Check sheet for the modelled part. Datum: model origin and axes. Units: mm. A direction names the side the tool comes from. Give positions to 0.01 mm unless a question says otherwise; leave off trailing zeros. Order: outer loops, then holes, each group sorted by start corner. A loop starts at its lowest first (then second) coordinate and runs counter-clockwise, first axis right, second up. Notation, with made-up numbers: M -34.5,87.25 L 8.5,87.25 A26 cw 8.5,109.25 Z; hole C 15.25,50 d7. An arc over 180 degrees is marked long. Return JSON: item names as keys, results as strings. Group by question number.
from build123d import *

# Parameters (mm, degrees)
BOSS_EXTRUDE2_DEPTH = 5.08
FILLET2_R           = 9.525
FILLET3_R           = 25.4


with BuildPart() as part:
    # Sketch5 → Boss-Extrude2 (new body)
    with BuildSketch(Plane(origin=(0, 0, -50.8), x_dir=(-1, 0, 0), z_dir=(0, 0, -1))):
        with BuildLine():
            Line((-52.084134713, -74.90469108), (-56.217901117, -96.079564574))
            ThreePointArc((-56.217901117, -96.079564574), (-56.227450796, -96.143111106), (-56.231425689, -96.207248133))
            Line((-56.231425689, -96.207248133), (-56.695270711, -121.603012501))
            Line((-56.695270711, -121.603012501), (-61.45697653, -121.516041559))
            Line((-61.45697653, -121.516041559), (-61.688899041, -134.213923743))
            Line((-61.688899041, -134.213923743), (-56.927193222, -134.300894684))
            Line((-56.927193222, -134.300894684), (-57.620624926, -172.266653317))
            Line((-57.620624926, -172.266653317), (-36.877249891, -96.432815008))
            Line((-36.877249891, -96.432815008), (19.109812826, -97.455399718))
            Line((19.109812826, -97.455399718), (37.101706355, -172.266653317))
            Line((37.101706355, -172.266653317), (37.763549432, -136.03038898))
            Line((37.763549432, -136.03038898), (42.525255251, -136.117359921))
            Line((42.525255251, -136.117359921), (42.757177762, -123.419477738))
            Line((42.757177762, -123.419477738), (37.995471943, -123.332506796))
            Line((37.995471943, -123.332506796), (38.459316965, -97.936742429))
            ThreePointArc((38.459316965, -97.936742429), (38.457686823, -97.872503028), (38.450464051, -97.808650153))
            Line((38.450464051, -97.808650153), (35.09270057, -76.496946406))
            Line((35.09270057, -76.496946406), (39.797167723, -75.755734526))
            Line((39.797167723, -75.755734526), (36.832320201, -56.937865912))
            Line((36.832320201, -56.937865912), (32.127853048, -57.679077792))
            Line((32.127853048, -57.679077792), (24.22159299, -7.498094822))
            ThreePointArc((24.22159299, -7.498094822), (23.977671585, -7.057207813), (23.507420242, -6.876258426))
            Line((23.507420242, -6.876258426), (11.818416858, -6.662762744))
            Line((11.818416858, -6.662762744), (11.905387799, -1.901056925))
            Line((11.905387799, -1.901056925), (-26.188258752, -1.205289392))
            Line((-26.188258752, -1.205289392), (-26.275229693, -5.966995211))
            Line((-26.275229693, -5.966995211), (-37.964233078, -5.753499529))
            ThreePointArc((-37.964233078, -5.753499529), (-38.44077853, -5.917155993), (-38.700637178, -6.348841631))
            Line((-38.700637178, -6.348841631), (-48.434089931, -56.20764123))
            Line((-48.434089931, -56.20764123), (-53.108352393, -55.295130035))
            Line((-53.108352393, -55.295130035), (-56.758397176, -73.992179884))
            Line((-56.758397176, -73.992179884), (-52.084134713, -74.90469108))
        make_face()
        Polygon((-31.935446416, -71.118839034), (-23.256774895, -26.66306829), (8.046213899, -27.234806762), (15.095699394, -71.977846959), align=None, mode=Mode.SUBTRACT)
    extrude(amount=BOSS_EXTRUDE2_DEPTH)

    # Fillet2
    fillet2_edges = [part.edges().sort_by_distance(p)[0] for p in [
        (31.935446416, -71.118839034, -53.34),
        (-15.095699394, -71.977846959, -53.34),
        (-8.046213899, -27.234806762, -53.34),
        (23.256774895, -26.66306829, -53.34),
    ]]
    fillet(fillet2_edges, radius=FILLET2_R)

    # Fillet3
    fillet3_edges = [part.edges().sort_by_distance(p)[0] for p in [
        (-19.109812826, -97.455399718, -53.34),
        (36.877249891, -96.432815008, -53.34),
    ]]
    fillet(fillet3_edges, radius=FILLET3_R)


solid = part.part
1) Release check for a two-part mould opening along X. For faces 1 (the face through (49.964, -144.275, -53.304)), 2 (the face through (10, -86, -50.8)), 3 (the face through (-38.335, -66.479, -53.304)) record: released by +X, released by -X, zero draft, split by the parting line, or undercut.
2) Sectioned sample at B-B on y = -52. Record the boundary of the cut face in (x, z), then the cut area to 3 significant figures.
3) Material ranges on line 1 along X through (y, z) = (-120.5, -53.05); line 2 along X through (y, z) = (-107.5, -51.95); line 3 along Y through (x, z) = (10, -51.9), recorded low to high.
4) Depth check by flat-ended pin: P1, Ø2, axis at x = 39.5, z = -52.5, coming from the -Y side; P2, Ø1, axis at x = -21.5, z = -55, coming from the +Y side. Enter the tip coordinate at first touch or a pass-through.
5) Sectioned sample at C-C on x = -30. Record the boundary of the cut face in (y, z).
6) Tool access check on faces 4 (the face through (-11.28, -47.77, -53.3)), 5 (the face through (-36.795, -87.302, -53.304)), 6 (the face through (50.739, -55.758, -53.304)), 7 (the face through (-30.31, -144.02, -53.3)). Record the directions out of +Z, -Z, +X, -X, +Y, -Y that give a thin tool (end or side, any length) a straight path to the whole face; none if there is none.
7) Sectioned sample at A-A on x = 2.5. Record the boundary of the cut face in (y, z), then the cut area to 3 significant figures.
Reply:
{
 "1": {"face 1": "undercut", "face 2": "zero draft", "face 3": "released by -X"},
 "2": {"outline": "M -31.23,-55.88 L -11.95,-55.88 L -11.95,-50.8 L -31.23,-50.8 Z; M 28.2,-55.88 L 47.61,-55.88 L 47.61,-50.8 L 28.2,-50.8 Z", "area": "197 mm^2"},
 "3": {"line 1": "-38.05 to -24.65, 43.46 to 56.68", "line 2": "-38.28 to -19.51, 38.31 to 56.44", "line 3": "-96.92 to -71.52, -26.91 to -1.5"},
 "4": {"P1": "y = -111.22", "P2": "y = -6.83"},
 "5": {"outline": "M -142.74,-55.88 L -44.17,-55.88 L -44.17,-50.8 L -142.74,-50.8 Z"},
 "6": {"face 4": "+Z, -Z", "face 5": "+Z, -Z, -X", "face 6": "+Z, -Z, +Y", "face 7": "+Z, -Z, -Y"},
 "7": {"outline": "M -97.06,-55.88 L -71.66,-55.88 L -71.66,-50.8 L -97.06,-50.8 Z; M -27.04,-55.88 L -1.64,-55.88 L -1.64,-50.8 L -27.04,-50.8 Z", "area": "258 mm^2"}
}
